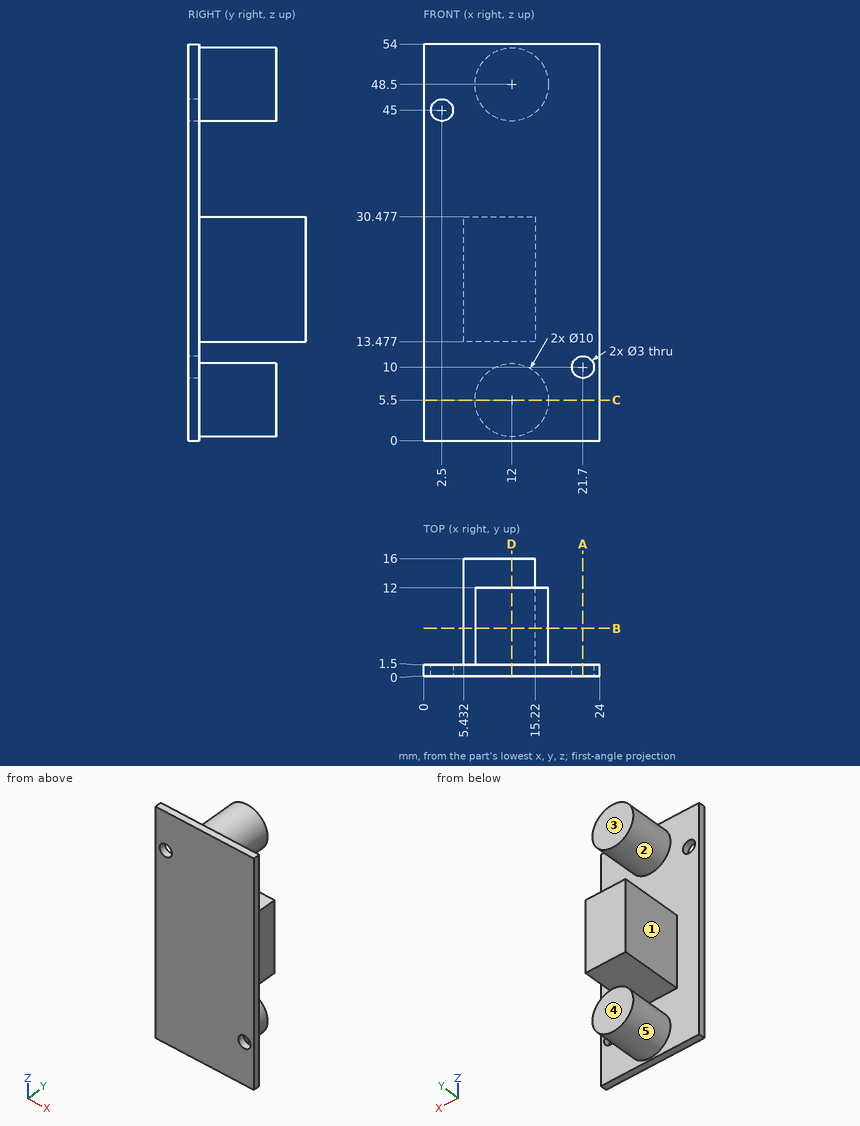
Print and shaded views of the part. All mm, measured from the part's lowest x, y and z. A direction names the side the tool comes from. Round coordinates to 2 decimals unless told otherwise and drop trailing zeros. Order: outer loops, then holes, each group sorted by start corner. A loop starts at its lowest first (then second) coordinate and runs counter-clockwise, first axis right, second up.
Q1. Wall check: L1, parallel to Z at x = 21.7, y = 0.9; L2, parallel to Z at x = 2.5, y = 0.5; L3, parallel to Y at x = 14.75, z = 46.5. Give the ranges that are in metal, low to high.
Q2. Slice it at D-D (x = 12). Write the cut outline in (y, z).
Q3. Two-plate mould, pull along Z, no slides. Class the marked faces 4 and 5: pulls with the +Z half, pulls with the -Z half, needs draft (parallel to the pull), parting line crosses it, or undercut.
Q4. Slice it at C-C (z = 5.5). Write the cut outline in (x, y), and give its area (3 significant figures).
Q5. Drop flat-ended pins along their axis: pin 1 (2 mm diameter, centred on x = 8.5, y = 11, fed in from -Z); pin 2 (1 mm diameter, centred on y = 2.5, z = 32, fed in from +X); pin 3 (11 mm diameter, centred on x = 13.5, z = 49, fed in from +Y); pin 4 (1 mm diameter, centred on x = 9, y = 9.5, fed in from +Z). Give the stop position or say it passes through.
Q6. Slice it at A-A (x = 21.7). Write the cut outline in (y, z).
Q7. Which spindle directions (+Z, -Z, +X, -X, +Y, -Y) get a long thin tool onto all of the face, cutting with end or side? Do the marked faces 1, 2 and 3. Say none if no direction does.
Q8. Slice it at B-B (y = 6.5). Write the cut outline in (x, z).
Results below:
1. L1: z = 0 to 8.5, 11.5 to 54
1. L2: z = 0 to 43.5, 46.5 to 54
1. L3: y = 0 to 12
2. outline: (0, 0) - (1.5, 0) - (1.5, 0.5) - (12, 0.5) - (12, 10.5) - (1.5, 10.5) - (1.5, 13.48) - (16, 13.48) - (16, 30.48) - (1.5, 30.48) - (1.5, 43.5) - (12, 43.5) - (12, 53.5) - (1.5, 53.5) - (1.5, 54) - (0, 54) - close
3. face 4: needs draft
3. face 5: undercut
4. outline: (0, 0) - (24, 0) - (24, 1.5) - (17, 1.5) - (17, 12) - (7, 12) - (7, 1.5) - (0, 1.5) - close
4. area: 141 mm2
5. pin 1: stops at z = 1.17
5. pin 2: passes through
5. pin 3: stops at y = 12
5. pin 4: stops at z = 52.83
6. outline: (0, 0) - (1.5, 0) - (1.5, 8.5) - (0, 8.5) - close; (0, 11.5) - (1.5, 11.5) - (1.5, 54) - (0, 54) - close
7. face 1: +Z, -Z, -X, +Y
7. face 2: +Y
7. face 3: +Z, +X, -X, +Y
8. outline: (5.43, 13.48) - (15.22, 13.48) - (15.22, 30.48) - (5.43, 30.48) - close; circle Ø10 at (12, 5.5); circle Ø10 at (12, 48.5)
